```python
from build123d import *

# Parameters (mm, degrees)
SKETCH_2_W           = 21
SKETCH_2_H           = 24
EXTRUDE_1_DEPTH      = 1
SKETCH_3_R           = 1.4
CUT_EXTRUDE_1_DEPTH  = 16.976545309
SKETCH_4_R           = 2.5
EXTRUDE_2_DEPTH      = 5
CHAMFER_1_SIZE       = 1
FILLET_3_R           = 2.5
SKETCH_5_W           = 6.518787968
SKETCH_5_H           = 1.296166803
EXTRUDE_3_DEPTH      = 3.5
EXTRUDE_4_DEPTH      = 3
EXTRUDE_4_DEPTH_BACK = 3
SKETCH_8_W           = 1.5
SKETCH_8_H           = 1.449096172
CUT_EXTRUDE_3_DEPTH  = 19.473018506


with BuildPart() as part:
    # Sketch 2 → Extrude 1 (new body)
    with BuildSketch(Plane.XY):
        Rectangle(SKETCH_2_W, SKETCH_2_H)
    extrude(amount=EXTRUDE_1_DEPTH)

    # Sketch 3 → Cut-Extrude 1 (cut, through all)
    with BuildSketch(Plane.XY.offset(1)):
        with Locations((7.375, 9.5)):
            Circle(SKETCH_3_R)
        with Locations(Location((-7.375, 9.5, 0), (0, 0, 180))):
            Circle(SKETCH_3_R)
    extrude(amount=-CUT_EXTRUDE_1_DEPTH, mode=Mode.SUBTRACT)

    # Sketch 4 → Extrude 2 (add)
    with BuildSketch(Plane.XY.offset(1)):
        with Locations((-5.400830934, -7.13462041)):
            Circle(SKETCH_4_R)
    extrude(amount=EXTRUDE_2_DEPTH)

    # Chamfer 1
    chamfer_1_edges = [part.edges().sort_by_distance(p)[0] for p in [
        (10.5, -12, 0.5),
        (-10.5, -12, 0.5),
        (-10.5, 12, 0.5),
        (10.5, 12, 0.5),
    ]]
    chamfer(chamfer_1_edges, length=CHAMFER_1_SIZE)

    # Fillet 3
    fillet_3_edges = [part.edges().sort_by_distance(p)[0] for p in [
        (-7.900830934, -7.13462041, 6),
    ]]
    fillet(fillet_3_edges, radius=FILLET_3_R)

    # Sketch 5 → Extrude 3 (add)
    with BuildSketch(Plane.XY.offset(1)):
        with Locations((0, 10.168737176)):
            Rectangle(SKETCH_5_W, SKETCH_5_H)
    extrude(amount=EXTRUDE_3_DEPTH)

    # Sketch 7 → Extrude 4 (add, two sides: drawn at the far end of the back side and taken through both)
    with BuildSketch(Plane(origin=(0, 0, 0), x_dir=(0, 0, -1), z_dir=(1, 0, 0)).offset(-EXTRUDE_4_DEPTH_BACK)):
        Polygon((-4.5, 10.48888975), (-5.626632975, 10.48888975), (-5.626632975, 13.964326433), (-5.949096172, 13.964326433), (-5.949096172, 10.168737175), (-4.5, 10.168737175), align=None)
    extrude(amount=EXTRUDE_4_DEPTH + EXTRUDE_4_DEPTH_BACK)

    # Sketch 8 → Cut-Extrude 3 (cut, through all)
    with BuildSketch(Plane(origin=(0, 0, 0), x_dir=(1, 0, 0), z_dir=(0, 1, 0))):
        with Locations((-1.28314556, -5.224548086)):
            Rectangle(SKETCH_8_W, SKETCH_8_H)
        with Locations((1.21685444, -5.224548086)):
            Rectangle(SKETCH_8_W, SKETCH_8_H)
    extrude(amount=CUT_EXTRUDE_3_DEPTH, mode=Mode.SUBTRACT)


solid = part.part
```
Check sheet for the modelled part. Datum: model origin and axes. Units: mm. A direction names the side the tool comes from. Coordinates: 2 decimals unless noted, no trailing zeros. Order: outer loops, then holes, each group sorted by start corner. A loop starts at its lowest first (then second) coordinate and runs counter-clockwise, first axis right, second up. Notation, with made-up numbers: (57.25, 61.25) -> (72.25, 61.25) arc R24 ccw to (72.25, 85.25) -> close; hole circle Ø3 at (-23.5, 54). An arc over 180 degrees is marked (long way). Write each question's results on one line, items separated by ' | '. Start each with the question number.
1) Section check D-D (x = 4). Enter the section's corners in (y, z), and give its area (3 significant figures).
2) Section check C-C (z = 2.9). Enter the section's corners in (x, y).
3) Material ranges on line 1 along Z through (x, y) = (0, 4.75); line 2 along Z through (x, y) = (-2.25, 11); line 3 along Y through (x, z) = (1.75, 0.85), recorded low to high.
4) Draft check along Z on faces 5 (the face through (-2.5, 10.489, 5.1)), 6 (the face through (0, 12, 5.949)), 7 (the face through (0, 9.521, 3)). Enter one of: pulls with the +Z half, pulls with the -Z half, needs draft (parallel to the pull), parting line crosses it, or undercut.
5) Set-up check for faces 1 (the face through (3.259, 10, 3)), 2 (the face through (-3.016, -6.384, 2.232)), 3 (the face through (-0.1, 12, 0.5)), 4 (the face through (2.5, 12.2, 5.627)): record each of +Z, -Z, +X, -X, +Y, -Y from which the full face is reachable in a straight line by a thin tool's end or side.
6) Section check B-B (x = 6.5). Enter the section's corners in (y, z).
7) Section check A-A (z = 0.65). Enter the section's corners in (x, y) (3 decimals).
8) Depth check by flat-ended pin: pin 1 (10.5 mm diameter, centred on x = 4.5, y = 0.5, fed in from +Z); pin 2 (1.1 mm diameter, centred on x = 2.5, z = 5, fed in from +Y); pin 3 (0.5 mm diameter, centred on x = -2.5, z = 5, fed in from -Y); pin 4 (1.5 mm diameter, centred on y = 7.5, z = 2.5, fed in from -X). Enter the tip coordinate at first touch or a pass-through.
Checked values:
1) outline: (-12, 0) -> (12, 0) -> (12, 1) -> (-12, 1) -> close | area: 24.0 mm²
2) outline: circle Ø5 at (-5.4, -7.13); (-3.26, 9.52) -> (3.26, 9.52) -> (3.26, 10.82) -> (-3.26, 10.82) -> close
3) line 1: 0 to 1 | line 2: 0 to 1, 5.63 to 5.95 | line 3: -12 to 12
4) face 5: undercut | face 6: pulls with the +Z half | face 7: needs draft
5) face 1: +Z, +X, +Y, -Y | face 2: +Z | face 3: -Z, +X, -X, +Y | face 4: +X, -X, +Y
6) outline: (-12, 0) -> (8.41, 0) -> (8.41, 1) -> (-12, 1) -> close; (10.59, 0) -> (12, 0) -> (12, 1) -> (10.59, 1) -> close
7) outline: (-10.5, -11) -> (-9.5, -12) -> (9.5, -12) -> (10.5, -11) -> (10.5, 11) -> (9.5, 12) -> (-9.5, 12) -> (-10.5, 11) -> close; hole circle Ø2.8 at (-7.375, 9.5); hole circle Ø2.8 at (7.375, 9.5)
8) pin 1: z = 1 | pin 2: y = 10.82 | pin 3: y = 10.17 | pin 4: through
